```python
from build123d import *

# Parameters (mm, degrees)
BOSS_EXTRUDE1_DEPTH = 135.3879
SKETCH2_R           = 3.2639
CUT_EXTRUDE1_DEPTH  = 1.6002


with BuildPart() as part:
    # Sketch1 → Boss-Extrude1 (new body)
    with BuildSketch(Plane(origin=(0, 0, 0), x_dir=(0, 0, -1), z_dir=(1, 0, 0))):
        Polygon((0, 0), (0, -1.6002), (55, -1.6002), (55, -89.49088), (0, -89.49088), (0, -91.09108), (56.6002, -91.09108), (56.6002, 0), align=None)
    extrude(amount=BOSS_EXTRUDE1_DEPTH)

    # Sketch2 → Cut-Extrude1 (cut)
    with BuildSketch(Plane.XY.offset(-55)):
        with Locations((67.69395, -32.84554)):
            Circle(SKETCH2_R)
        with Locations((67.69395, -58.24554)):
            Circle(SKETCH2_R)
        with Locations((54.99395, -45.54554)):
            Circle(SKETCH2_R)
        with Locations((80.39395, -45.54554)):
            Circle(SKETCH2_R)
    extrude(amount=-CUT_EXTRUDE1_DEPTH, mode=Mode.SUBTRACT)


solid = part.part
```
The listing builds one solid part. Answer for the finished solid, in the listing's coordinates (mm). A direction names the side the tool comes from. Give positions to 0.01 mm unless a question says otherwise; leave off trailing zeros. Write each loop counter-clockwise with the first axis right and the second up, starting at its lowest first coordinate (ties: lowest second). Pieces come first, ordered by that corner, then holes. Notation, with made-up numbers: (-17.5, 39.25) -> (41.5, 39.25) arc R26 cw to (41.5, 63.25) -> close; hole circle Ø5 at (-24, -28.5). An arc over 180 degrees is marked (long way). Write item = value, one per line. Start each with the question number.
1) The part is cut by section A-A, the plane z = -23. Determine the outline of the cut face in (x, y), and give its area (3 significant figures).
2) The part is cut by section C-C, the plane y = -47. Determine the outline of the cut face in (x, z), and give its area (3 significant figures).
3) The part is cut by section D-D, the plane x = 119. Determine the outline of the cut face in (y, z).
4) Straight lines are drawn through the part: line 1 along Y through (x, z) = (37, -23.5); line 2 along Z through (x, y) = (112.5, -14.5). For each, find the intervals that lie inside material, in ascending order.
5) Which of the six approach directions +Z, -Z, +X, -X, +Y, -Y give full straight-line access (tool end or side, diameter ignored) to faces 1 (the face through (135.388, -25.1, -55.4)), 2 (the face through (67, -1.6, -27))?
6) Determine the mould class of faces 3 (the face through (67, 0, -29)), 4 (the face through (67, -91.091, -28)), 5 (the face through (64.433, -32.702, -55.789)) for opening direction Y: +Y half, -Y half, draft (parallel to the pull), parting line (faces both ways), or undercut.
7) The part is cut by section B-B, the plane x = 67. Determine the outline of the cut face in (y, z), and give its area (3 significant figures).
8) Each of these flat-tipped pins is pushed along its axis until it touches: pin 1 (8.5 mm diameter, centred on x = 54.99, y = -45.55, fed in from +Z); pin 2 (5 mm diameter, centred on x = 80.39, y = -45.55, fed in from -Z). Where does it stop, or does it pass through?
Solutions:
q1.outline = (0, -91.09) -> (135.39, -91.09) -> (135.39, -89.49) -> (0, -89.49) -> close; (0, -1.6) -> (135.39, -1.6) -> (135.39, 0) -> (0, 0) -> close
q1.area = 433 mm²
q2.outline = (0, -56.6) -> (52.07, -56.6) -> (52.07, -55) -> (0, -55) -> close; (57.92, -56.6) -> (77.47, -56.6) -> (77.47, -55) -> (57.92, -55) -> close; (83.32, -56.6) -> (135.39, -56.6) -> (135.39, -55) -> (83.32, -55) -> close
q2.area = 198 mm²
q3.outline = (-91.09, -56.6) -> (0, -56.6) -> (0, 0) -> (-1.6, 0) -> (-1.6, -55) -> (-89.49, -55) -> (-89.49, 0) -> (-91.09, 0) -> close
q4.line_1 = -91.09 to -89.49, -1.6 to 0
q4.line_2 = -56.6 to -55
q5.face_1 = +Z, -Z, +X, +Y, -Y
q5.face_2 = +Z, +X, -X
q6.face_3 = +Y half
q6.face_4 = -Y half
q6.face_5 = undercut
q7.outline = (-91.09, -56.6) -> (-61.43, -56.6) -> (-61.43, -55) -> (-89.49, -55) -> (-89.49, 0) -> (-91.09, 0) -> close; (-55.06, -56.6) -> (-36.03, -56.6) -> (-36.03, -55) -> (-55.06, -55) -> close; (-29.66, -56.6) -> (0, -56.6) -> (0, 0) -> (-1.6, 0) -> (-1.6, -55) -> (-29.66, -55) -> close
q7.area = 301 mm²
q8.pin_1 = -55
q8.pin_2 = through
